The listing builds one solid part. Answer for the finished solid, in the listing's coordinates (mm). A direction names the side the tool comes from. Coordinates: 2 decimals unless noted, no trailing zeros. Order: outer loops, then holes, each group sorted by start corner. A loop starts at its lowest first (then second) coordinate and runs counter-clockwise, first axis right, second up.
```python
from build123d import *

# Parameters (mm, degrees)
F0_W     = 213
F0_H     = 200
F1_DEPTH = 25
F3_DEPTH = 50
F5_DEPTH = 25
F6_R     = 5
F7_DEPTH = 45
F8_R     = 5
F9_R     = 10


with BuildPart() as f1:
    # F0 (on Top) → F1 (new body)
    with BuildSketch(Plane.XY):
        with Locations((-106.5, 100)):
            Rectangle(F0_W, F0_H)
    extrude(amount=F1_DEPTH)

    # F2 (on face) → F3 (cut)
    with BuildSketch(Plane.XY.offset(25)):
        Polygon((0, 160), (0, 200), (-40, 200), align=None)
        Polygon((-213, 40), (-213, 0), (-173, 0), align=None)
    extrude(amount=-F3_DEPTH, mode=Mode.SUBTRACT)

    # F4 (on face) → F5 (join)
    with BuildSketch(Plane.XY.offset(25)):
        with BuildLine():
            ThreePointArc((-184.1421356237, 116.1421356237), (-184.1421356237, 87.8578643763), (-155.8578643763, 87.8578643763))
            Line((-155.8578643763, 87.8578643763), (-87.8578643763, 155.8578643763))
            ThreePointArc((-87.8578643763, 155.8578643763), (-87.8578643763, 184.1421356237), (-116.1421356237, 184.1421356237))
            Line((-116.1421356237, 184.1421356237), (-184.1421356237, 116.1421356237))
        make_face()
        with BuildLine():
            Line((-94.9289321881, 162.9289321881), (-162.9289321881, 94.9289321881))
            ThreePointArc((-162.9289321881, 94.9289321881), (-177.0710678119, 94.9289321881), (-177.0710678119, 109.0710678119))
            Line((-177.0710678119, 109.0710678119), (-109.0710678119, 177.0710678119))
            ThreePointArc((-109.0710678119, 177.0710678119), (-94.9289321881, 177.0710678119), (-94.9289321881, 162.9289321881))
        make_face(mode=Mode.SUBTRACT)
        with BuildLine():
            ThreePointArc((-59.4369521161, 142.218487395), (-89.3898269447, 89.3898269447), (-142.218487395, 59.4369521161))
            ThreePointArc((-142.218487395, 59.4369521161), (-144.9428693216, 57.6623958613), (-146, 54.58769563))
            Line((-146, 54.58769563), (-146, 14))
            ThreePointArc((-146, 14), (-144.5355339059, 10.4644660941), (-141, 9))
            Line((-141, 9), (-74, 9))
            ThreePointArc((-74, 9), (-70.4644660941, 10.4644660941), (-69, 14))
            Line((-69, 14), (-69, 34.554946274))
            ThreePointArc((-69, 34.554946274), (-61.9705627485, 51.5255090224), (-45, 58.554946274))
            Line((-45, 58.554946274), (-14, 58.554946274))
            ThreePointArc((-14, 58.554946274), (-10.4644660941, 60.019412368), (-9, 63.554946274))
            Line((-9, 63.554946274), (-9, 141))
            ThreePointArc((-9, 141), (-10.4644660941, 144.5355339059), (-14, 146))
            Line((-14, 146), (-54.58769563, 146))
            ThreePointArc((-54.58769563, 146), (-57.6623958613, 144.9428693216), (-59.4369521161, 142.218487395))
        make_face()
    extrude(amount=F5_DEPTH)

    # F6
    f6_edges = [f1.edges().sort_by_distance(p)[0] for p in [
        (-121.857864, 121.857864, 25),
    ]]
    fillet(f6_edges, radius=F6_R)

    # F7 (cut): a face of the model
    f7_faces = [f1.faces().sort_by_distance(p)[0] for p in [
        (-71.1078293712, 72.4638953315, 50),
    ]]
    extrude(f7_faces, amount=-F7_DEPTH, mode=Mode.SUBTRACT)

    # F8
    f8_edges = [f1.edges().sort_by_distance(p)[0] for p in [
        (-146, 34.293848, 25),
        (-89.389827, 89.389827, 5),
    ]]
    fillet(f8_edges, radius=F8_R)

    # F9
    f9_edges = [f1.edges().sort_by_distance(p)[0] for p in [
        (0, 0, 12.5),
        (-213, 200, 12.5),
    ]]
    fillet(f9_edges, radius=F9_R)


solid = f1.part
```
1) A cutting plane is placed at B-B, the plane x = -35.5. Write down the section's boundary in (y, z).
2) Each of these flat-tipped pins is pushed along its axis until it touches: P1, Ø1.5, axis at y = 166, z = 40.5, coming from the -X side; P2, Ø1.5, axis at x = -100.5, y = 101, coming from the -Z side; P3, Ø3, axis at x = -152, z = 33, coming from the -Y side; P4, Ø10, axis at x = -30, y = 50.5, coming from the +Z side. Where does it stop, or does it pass through?
3) The mould has two halves that part along Y. Classify faces 1 (the cylindrical face through (-151.681, 150.729, 26.426)), 2 (the flat face through (-128, 128, 50)), 3 (the cylindrical face through (-107, 10, 7)), 4 (the cylindrical face through (-120.319, 121.271, 26.426)): released by +Y, released by -Y, zero draft, split by the parting line, or undercut.
4) A cutting plane is placed at C-C, the plane y = 24. Write down the section's boundary in (x, z).
5) For faces 5 (the cylindrical face through (-176.914, 94.775, 37.325)), 6 (the flat face through (0, 84, 12)), 7 (the flat face through (-149.666, 150.618, 39.86)), determine the directions among +Z, -Z, +X, -X, +Y, -Y from which every point of the face is accessible in a straight line to the end or side of a thin tool.
6) Straight lines are drawn through the part: probe 1 along Z at (x, y) = (-197, 56.5); probe 2 along X at (y, z) = (168, 35.5); probe 3 along Y at (x, z) = (-127, 35). For each, find the intervals that lie inside material, in ascending order.
Working result:
1. outline: (0, 0) - (195.5, 0) - (195.5, 25) - (151, 25) arc R5 ccw to (146, 20) - (146, 10) arc R5 cw to (141, 5) - (63.55, 5) arc R5 cw to (58.55, 10) - (58.55, 20) arc R5 ccw to (53.55, 25) - (0, 25) - close
2. P1: stops at x = -135.03
2. P2: stops at z = 0
2. P3: stops at y = 90.22
2. P4: stops at z = 25
3. face 1: released by +Y
3. face 2: zero draft
3. face 3: undercut
3. face 4: released by -Y
4. outline: (-197, 0) - (0, 0) - (0, 25) - (-64, 25) arc R5 ccw to (-69, 20) - (-69, 10) arc R5 cw to (-74, 5) - (-141, 5) arc R5 cw to (-146, 10) - (-146, 20) arc R5 ccw to (-151, 25) - (-197, 25) - close
5. face 5: +Z
5. face 6: +Z, -Z, +X, +Y, -Y
5. face 7: +Z, -X, +Y
6. probe 1: z = 0 to 25
6. probe 2: x = -132.28 to -118.14, -92.2 to -82.1
6. probe 3: y = 116.72 to 130.86, 159.14 to 173.28
